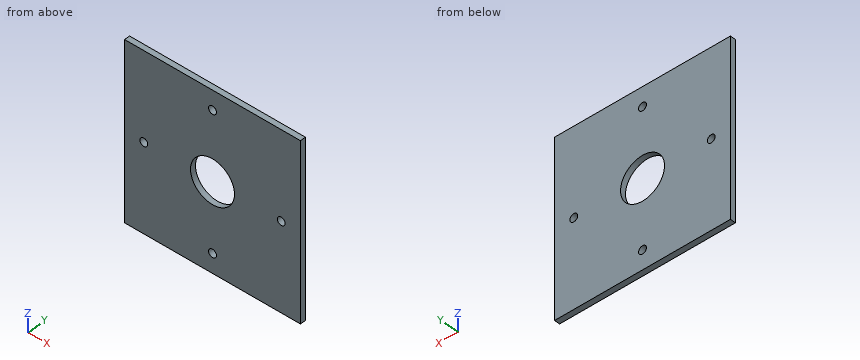
Autodesk Inventor part; units mm, degrees
ref_plane "YZ Plane" through (0, 0, 0) normal (1, 0, 0) x (0, 1, 0)
ref_plane "XZ Plane" through (0, 0, 0) normal (0, 1, 0) x (-1, 0, 0)
ref_plane "XY Plane" through (0, 0, 0) normal (0, 0, 1) x (1, 0, 0)
sketch "Sketch1" plane through (0, 0, 0) normal (0, 1, 0) x (-1, 0, 0)
  line L0 (0, 0) -> (101.6, 0)
  line L1 (101.6, 0) -> (101.6, -101.6)
  line L2 (101.6, -101.6) -> (0, -101.6)
  line L3 (0, -101.6) -> (0, 0)
  circle A0 centre (90.4875, -50.8) radius 2.286
  circle A1 centre (50.8, -50.8) radius 12.7
  circle A2 centre (50.8, -90.4875) radius 2.286
  circle A3 centre (11.1125, -50.8) radius 2.286
  circle A4 centre (50.8, -11.1125) radius 2.286
  point P0 (101.6, -50.8)
  point P1 (50.8, -101.6)
  dimension "d0" = 101.6
  dimension "d1" = 101.6
  dimension "d2" = 4.572
  dimension "d3" = 11.1125
  dimension "d4" = 25.4
  dimension "d7" = 360
extrude "Extrusion1" add sketch "Sketch1" along normal blind 3.175
properties part number "Top plate" material "Acetal Resin, White"
Build history of the part. All positions in model axes, mm. Give positions to 0.01 mm unless a question says otherwise; leave off trailing zeros. Order: outer loops, then holes, each group sorted by start corner. A loop starts at its lowest first (then second) coordinate and runs counter-clockwise, first axis right, second up. Notation, with made-up numbers: M 27,-39 L 63,-39 A13 ccw 63,-33 Z; hole C 51,5 d5. An arc over 180 degrees is marked long. Write item = value, one per line. Start each with the question number.
(1) Slice it at A-A on x = -50.8. Write the cut outline in (y, z) (1 decimal).
(2) Slice it at B-B on z = -50.8. Write the cut outline in (x, y) (1 decimal).
(3) Slice it at C-C on y = 2.4. Write the cut outline in (x, z), plus the area to 3 significant figures.
(4) Pin check, flat tip, straight feed: pin 1 Ø3.5 at (x, z) = (-50.8, -90.49) entering from -Y. Stop position of the tip, or through.
(5) Probe L1, parallel to Z at x = -50.8, y = 2.1; L2, parallel to X at y = 0.85, z = -92.5; L3, parallel to Z at x = -54.5, y = 2.25. List the from-to ranges inside material, lowest first. Write a range as [from, to].
Responses:
q1.outline = M 0,-101.6 L 3.2,-101.6 L 3.2,-92.8 L 0,-92.8 Z; M 0,-88.2 L 3.2,-88.2 L 3.2,-63.5 L 0,-63.5 Z; M 0,-38.1 L 3.2,-38.1 L 3.2,-13.4 L 0,-13.4 Z; M 0,-8.8 L 3.2,-8.8 L 3.2,0 L 0,0 Z
q2.outline = M -101.6,0 L -92.8,0 L -92.8,3.2 L -101.6,3.2 Z; M -88.2,0 L -63.5,0 L -63.5,3.2 L -88.2,3.2 Z; M -38.1,0 L -13.4,0 L -13.4,3.2 L -38.1,3.2 Z; M -8.8,0 L 0,0 L 0,3.2 L -8.8,3.2 Z
q3.outline = M -101.6,-101.6 L 0,-101.6 L 0,0 L -101.6,0 Z; hole C -90.49,-50.8 d4.57; hole C -50.8,-50.8 d25.4; hole C -50.8,-90.49 d4.57; hole C -50.8,-11.11 d4.57; hole C -11.11,-50.8 d4.57
q3.area = 9,750 mm2
q4.pin_1 = through
q5.L1 = [-101.6, -92.77], [-88.2, -63.5], [-38.1, -13.4], [-8.83, 0]
q5.L2 = [-101.6, -51.88], [-49.72, 0]
q5.L3 = [-101.6, -62.95], [-38.65, 0]
